Verification items for the finished model (mm, model axes). A direction names the side the tool comes from. Coordinates: 2 decimals unless noted, no trailing zeros. Order: outer loops, then holes, each group sorted by start corner. A loop starts at its lowest first (then second) coordinate and runs counter-clockwise, first axis right, second up. Notation, with made-up numbers: (-29.5, -2.5) -> (26.5, -2.5) arc R22 ccw to (26.5, 35.5) -> close; hole circle Ø6 at (-20, 19.5). An arc over 180 degrees is marked (long way). Write each question's results on one line, items separated by ' | '. Start each with the question number.
(1) Go/stop test with flat-tipped pins: pin 1 (12 mm diameter, centred on x = 38, z = 12.5, fed in from -Y); pin 2 (10 mm diameter, centred on x = -12, z = 9.5, fed in from -Y) (3 decimals); pin 3 (10 mm diameter, centred on x = 11.5, z = 6, fed in from +Y) (3 decimals). Record where each tip stops, or that it passes through.
(2) Set-up check for faces 1 (the flat face through (-7.501, 0, 2)), 2 (the flat face through (-11, -3.175, 6)), 3 (the cylindrical face through (-0.03, 3.81, 8)), 4 (the flat face through (3, 3, -3.175)): record each of +Z, -Z, +X, -X, +Y, -Y from which the full face is reachable in a straight line by a thin tool's end or side.
(3) Cross-section at A-A on z = -6.5. Enter the section's corners in (x, y) (3 decimals), and give its area (3 significant figures).
(4) Cross-section at C-C on z = 5. Enter the section's corners in (x, y) (3 decimals).
(5) Cross-section at B-B on x = -1. Enter the section's corners in (y, z) (3 decimals), and give its area (3 significant figures).
(6) Cross-section at D-D on x = 32.5. Enter the section's corners in (y, z).
(7) Thickness scan on probe 1 along Z at (x, y) = (-12.5, 3) (3 decimals); probe 2 along Z at (x, y) = (16.5, 2); probe 3 along Y at (x, z) = (18.5, 8.5) (3 decimals). Record the ranges inside material, lowest first. Write a range as [from, to].
```python
from build123d import *

# Parameters (mm, degrees)
F1_DEPTH = 12.7
F3_DEPTH = 15.875
F4_DEPTH = 3.175
F6_DEPTH = 6.349999961
F7_W     = 12.7
F7_H     = 3.175
F8_DEPTH = 9.526


with BuildPart() as f1:
    # F0 (on Top) → F1 (new body)
    with BuildSketch(Plane.XY):
        with BuildLine():
            ThreePointArc((2.1060567419, -3.175), (3.3570951868, -1.8016692001), (3.81, 0))
            ThreePointArc((3.81, 0), (3.3570951868, 1.8016692001), (2.1060567419, 3.175))
            ThreePointArc((2.1060567419, 3.175), (0, 3.81), (-2.1060567419, 3.175))
            ThreePointArc((-2.1060567419, 3.175), (-3.81, 0), (-2.1060567419, -3.175))
            ThreePointArc((-2.1060567419, -3.175), (0, -3.81), (2.1060567419, -3.175))
        make_face()
        with BuildLine():
            ThreePointArc((2.1060567419, 3.175), (3.3570951868, 1.8016692001), (3.81, 0))
            ThreePointArc((3.81, 0), (3.3570951868, -1.8016692001), (2.1060567419, -3.175))
            Line((2.1060567419, -3.175), (21.7762735865, -3.175))
            Line((21.7762735865, -3.175), (46.5216673911, -19.1860459745))
            Line((46.5216673911, -19.1860459745), (49.9712098046, -13.8547087462))
            Line((49.9712098046, -13.8547087462), (23.6514521839, 3.175))
            Line((23.6514521839, 3.175), (2.1060567419, 3.175))
        make_face()
        with BuildLine():
            ThreePointArc((-2.1060567419, -3.175), (-3.81, 0), (-2.1060567419, 3.175))
            Line((-2.1060567419, 3.175), (-20.2012713999, 3.175))
            Line((-20.2012713999, 3.175), (-20.2012713999, -3.175))
            Line((-20.2012713999, -3.175), (-2.1060567419, -3.175))
        make_face()
    extrude(amount=F1_DEPTH)

    # F2 (on face) → F3 (join)
    with BuildSketch(Plane(origin=(0, 0, 0), x_dir=(1, 0, 0), z_dir=(0, 0, -1))):
        with BuildLine():
            ThreePointArc((2.1060567419, -3.175), (3.3570951868, -1.8016692001), (3.81, 0))
            ThreePointArc((3.81, 0), (3.3570951868, 1.8016692001), (2.1060567419, 3.175))
            ThreePointArc((2.1060567419, 3.175), (0, 3.81), (-2.1060567419, 3.175))
            ThreePointArc((-2.1060567419, 3.175), (-3.81, 0), (-2.1060567419, -3.175))
            ThreePointArc((-2.1060567419, -3.175), (0, -3.81), (2.1060567419, -3.175))
        make_face()
    extrude(amount=F3_DEPTH)

    # F2 (on face) → F4 (join, symmetric)
    with BuildSketch(Plane(origin=(0, 0, 0), x_dir=(1, 0, 0), z_dir=(0, 0, -1))):
        with BuildLine():
            ThreePointArc((2.1060567419, 3.175), (3.3570951868, 1.8016692001), (3.81, 0))
            ThreePointArc((3.81, 0), (3.3570951868, -1.8016692001), (2.1060567419, -3.175))
            Line((2.1060567419, -3.175), (5.499261314, -3.175))
            ThreePointArc((5.499261314, -3.175), (6.1336289969, -1.6435009364), (6.35, 0))
            ThreePointArc((6.35, 0), (6.1336289969, 1.6435009364), (5.499261314, 3.175))
            Line((5.499261314, 3.175), (2.1060567419, 3.175))
        make_face()
        with BuildLine():
            ThreePointArc((-2.1060567419, 3.175), (0, 3.81), (2.1060567419, 3.175))
            Line((2.1060567419, 3.175), (5.499261314, 3.175))
            ThreePointArc((5.499261314, 3.175), (0, 6.35), (-5.499261314, 3.175))
            Line((-5.499261314, 3.175), (-2.1060567419, 3.175))
        make_face()
        with BuildLine():
            Line((5.499261314, -3.175), (2.1060567419, -3.175))
            ThreePointArc((2.1060567419, -3.175), (0, -3.81), (-2.1060567419, -3.175))
            Line((-2.1060567419, -3.175), (-5.499261314, -3.175))
            ThreePointArc((-5.499261314, -3.175), (0, -6.35), (5.499261314, -3.175))
        make_face()
        with BuildLine():
            ThreePointArc((-2.1060567419, -3.175), (-3.81, 0), (-2.1060567419, 3.175))
            Line((-2.1060567419, 3.175), (-5.499261314, 3.175))
            ThreePointArc((-5.499261314, 3.175), (-6.35, 0), (-5.499261314, -3.175))
            Line((-5.499261314, -3.175), (-2.1060567419, -3.175))
        make_face()
    extrude(amount=F4_DEPTH, both=True)

    # F5 (on face) → F6 (join, through all)
    with BuildSketch(Plane(origin=(4.9781873283, 7.6938887107, 0), x_dir=(0.839580671, -0.5432350291, 0), z_dir=(-0.5432350291, -0.839580671, 0))):
        with BuildLine():
            ThreePointArc((42.3817091402, 0), (52.8799553739, -2.5479917191), (59.0062249688, 6.35))
            ThreePointArc((59.0062249688, 6.35), (52.8799553739, 15.2479917191), (42.3817091402, 12.7))
            Line((42.3817091402, 12.7), (49.4812249688, 12.7))
            Line((49.4812249688, 12.7), (49.4812249688, 0))
            Line((49.4812249688, 0), (42.3817091402, 0))
        make_face()
        with BuildLine():
            Line((49.4812249688, 12.7), (42.3817091402, 12.7))
            ThreePointArc((42.3817091402, 12.7), (39.9562249688, 6.35), (42.3817091402, 0))
            Line((42.3817091402, 0), (49.4812249688, 0))
            Line((49.4812249688, 0), (49.4812249688, 12.7))
        make_face()
    extrude(amount=-F6_DEPTH)

    # F7 (on face) → F8 (cut, through all)
    with BuildSketch(Plane.XZ.offset(3.175)):
        with Locations((-13.8512713999, 11.1125)):
            Rectangle(F7_W, F7_H)
        with Locations((-13.8512713999, 1.5875)):
            Rectangle(F7_W, F7_H)
    extrude(amount=-F8_DEPTH, mode=Mode.SUBTRACT)


solid = f1.part
```
Results are:
1) pin 1: stops at y = -17.55 | pin 2: stops at y = -3.175 | pin 3: stops at y = 3.175
2) face 1: -Z, -X, +Y, -Y | face 2: +Z, -X, -Y | face 3: +Z, +Y | face 4: -Z
3) outline: circle Ø7.62 at (0, 0) | area: 45.6 mm2
4) outline: (-20.201, -3.175) -> (-2.106, -3.175) arc R3.81 ccw to (2.106, -3.175) -> (21.776, -3.175) -> (54.438, -24.308) -> (57.887, -18.977) -> (23.651, 3.175) -> (2.106, 3.175) arc R3.81 ccw to (-2.106, 3.175) -> (-20.201, 3.175) -> close
5) outline: (-6.271, -3.175) -> (-3.676, -3.175) -> (-3.676, -15.875) -> (3.676, -15.875) -> (3.676, -3.175) -> (6.271, -3.175) -> (6.271, 3.175) -> (3.676, 3.175) -> (3.676, 12.7) -> (-3.676, 12.7) -> (-3.676, 3.175) -> (-6.271, 3.175) -> close | area: 243 mm2
6) outline: (-10.11, 0) -> (-2.55, 0) -> (-2.55, 12.7) -> (-10.11, 12.7) -> close
7) probe 1: z = [3.175, 9.525] | probe 2: z = [0, 12.7] | probe 3: y = [-3.175, 3.175]
